Here's how the part is built. I have some questions about the finished solid (model axes, mm). A direction names the side the tool comes from. Round coordinates to 2 decimals unless told otherwise and drop trailing zeros. Loops run counter-clockwise (first coordinate to the right, second up) from the corner with the lowest first, then second, coordinate; pieces in that order, holes last. Notation, with made-up numbers: M 31.5,28.25 L 81.5,28.25 A26 ccw 81.5,50.25 Z; hole C 45,16 d8. An arc over 180 degrees is marked long. Answer as a JSON object with one key per item and string values.
from build123d import *

# Parameters (mm, degrees)
SKETCH_1_R          = 15
SKETCH_1_W          = 10
SKETCH_1_H          = 10
EXTRUDE_1_DEPTH     = 80
SKETCH1_R           = 19
SKETCH1_W           = 10
SKETCH1_H           = 10
BOSS_EXTRUDE1_DEPTH = 3
CHAMFER1_SIZE       = 1
CHAMFER1_SIZE2      = 2.747477419


with BuildPart() as part:
    # Эскиз1 → Бобышка-Вытянуть1 (new body)
    with BuildSketch(Plane(origin=(0, 0, 0), x_dir=(1, 0, 0), z_dir=(0, 1, 0))):
        Circle(SKETCH_1_R)
        Rectangle(SKETCH_1_W, SKETCH_1_H, mode=Mode.SUBTRACT)
    extrude(amount=EXTRUDE_1_DEPTH)

    # Sketch1 → Boss-Extrude1 (add)
    with BuildSketch(Plane(origin=(0, 80, 0), x_dir=(1, 0, 0), z_dir=(0, 1, 0))):
        Circle(SKETCH1_R)
        Rectangle(SKETCH1_W, SKETCH1_H, mode=Mode.SUBTRACT)
    extrude(amount=-BOSS_EXTRUDE1_DEPTH)

    # Chamfer1
    chamfer1_edges = [part.edges().sort_by_distance(p)[0] for p in [
        (0, 80, -5),
        (-5, 80, 0),
        (0, 80, 5),
        (5, 80, 0),
    ]]
    chamfer1_side = [part.faces().sort_by_distance(p)[0] for p in [
        (-18.462598846, 80, 0),
    ]]
    chamfer(chamfer1_edges, length=CHAMFER1_SIZE, length2=CHAMFER1_SIZE2, reference=chamfer1_side[0])


solid = part.part
Item 1: I want a section at A-A, the plane z = 0. Please give me the cut outline in (x, y), then the cut area to 3 significant figures.
Resolved:
{"outline": "M -19,77 L -15,77 L -15,0 L -5,0 L -5,77.25 L -6,80 L -19,80 Z; M 5,0 L 15,0 L 15,77 L 19,77 L 19,80 L 6,80 L 5,77.25 Z", "area": "1,620 mm²"}
Item 2: I want a section at D-D, the plane z = -11.5. Please give me the cut outline in (x, y), then the cut area to 3 significant figures.
Resolved:
{"outline": "M -15.12,77 L -9.63,77 L -9.63,0 L 9.63,0 L 9.63,77 L 15.12,77 L 15.12,80 L -15.12,80 Z", "area": "1,570 mm²"}
Item 3: On a 3-axis mill with a long thin cutter (end or side, diameter ignored), from which of +Z, -Z, +X, -X, +Y, -Y can I reach the whole of each face in a straight line? I mean faces 1 (the face through (-0.084, 78.607, -5.493)), 2 (the face through (-14.985, 37.961, -0.66)), 3 (the face through (0, 38, -5)). Say none if no direction works.
Resolved:
{"face 1": "+Y", "face 2": "-Y", "face 3": "+Y, -Y"}
Item 4: Please list where these lines run through material, in increasing order: probe 1 along Z at (x, y) = (0, 4); probe 2 along Y at (x, z) = (-15, -3.5); probe 3 along Z at (x, y) = (-4.5, 19). Write a range as from..to.
Resolved:
{"probe 1": "-15..-5, 5..15", "probe 2": "77..80", "probe 3": "-14.31..-5, 5..14.31"}
Item 5: I want a section at B-B, the plane x = 0. Please give me the cut outline in (y, z).
Resolved:
{"outline": "M 0,-15 L 77,-15 L 77,-19 L 80,-19 L 80,-6 L 77.25,-5 L 0,-5 Z; M 0,5 L 77.25,5 L 80,6 L 80,19 L 77,19 L 77,15 L 0,15 Z"}
Item 6: I want a section at C-C, the plane y = 35. Please give me the cut outline in (x, z).
Resolved:
{"outline": "C 0,0 d30; hole M -5,-5 L 5,-5 L 5,5 L -5,5 Z"}
Item 7: I'm going to push flat-ended pins straight in: pin 1 Ø1.5 at (x, y) = (5, 31) entering from -Z; pin 2 Ø10 at (x, y) = (-10.5, 41) entering from +Z; pin 3 Ø11 at (y, z) = (33.5, -2) entering from +X. Where does each tip first touch, or does it pass through?
Resolved:
{"pin 1": "z = -14.39", "pin 2": "z = 13.96", "pin 3": "x = 15"}
